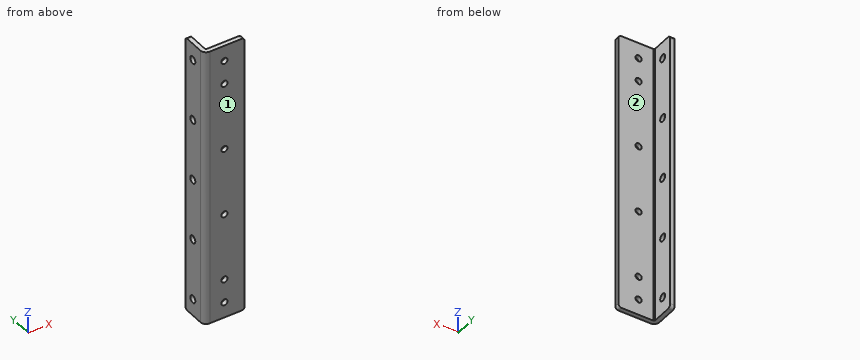
```python
from build123d import *

# Parameters (mm, degrees)
BASE_FLANGE1_START   = -125
BASE_FLANGE1_DEPTH   = 250
FILLET1_R            = 3
M5_CLEARANCE_HOLE1_D = 5.5
M5_CLEARANCE_HOLE2_D = 5.5
M6_CLEARANCE_HOLE1_D = 6.6


# Read off the part's stored shape, not the designer's step: Base-Flange1
with BuildPart() as part:
    # Base-Flange1 outline → Base-Flange1 (new body)
    with BuildSketch(Plane.XY.offset(BASE_FLANGE1_START)):
        with BuildLine():
            Line((5, 0), (36, 0))
            Line((36, 0), (36, 4))
            Line((36, 4), (5, 4))
            ThreePointArc((5, 4), (4.292893219, 4.292893219), (4, 5))
            Line((4, 5), (4, 25))
            Line((4, 25), (0, 25))
            Line((0, 25), (0, 5))
            ThreePointArc((0, 5), (1.464466094, 1.464466094), (5, 0))
        make_face()
    extrude(amount=BASE_FLANGE1_DEPTH)

    # Fillet1
    fillet1_edges = [part.edges().sort_by_distance(p)[0] for p in [
        (2, 25, 125),
        (2, 25, -125),
        (36, 2, 125),
        (36, 2, -125),
    ]]
    fillet(fillet1_edges, radius=FILLET1_R)

    # M5 Clearance Hole1 (through all)
    with Locations(Plane(origin=(0, 4, 0), x_dir=(1, 0, 0), z_dir=(0, 1, 0))):
        with Locations((18, 90), (18, 30), (18, -30), (18, -90)):
            Hole(M5_CLEARANCE_HOLE1_D / 2)

    # M5 Clearance Hole2 (through all)
    with Locations(Plane(origin=(0, 4, 0), x_dir=(1, 0, 0), z_dir=(0, 1, 0))):
        with Locations((18, -111), (18, 111)):
            Hole(M5_CLEARANCE_HOLE2_D / 2)

    # M6 Clearance Hole1 (through all)
    with Locations(Plane(origin=(4, 0, 0), x_dir=(0, 0, -1), z_dir=(1, 0, 0))):
        with Locations((-110, 15), (-55, 15), (0, 15), (55, 15), (110, 15)):
            Hole(M6_CLEARANCE_HOLE1_D / 2)


solid = part.part
```
Design review of the part built by this model. Coordinates are the model's own, in mm. Face numbers are marked on the shaded views. A direction names the side the tool comes from. Coordinates: 2 decimals unless noted, no trailing zeros. Order: outer loops, then holes, each group sorted by start corner. A loop starts at its lowest first (then second) coordinate and runs counter-clockwise, first axis right, second up. Notation, with made-up numbers: (58.25, 39.5) -> (67.25, 39.5) arc R20 cw to (67.25, 58.5) -> close; hole circle Ø4 at (5, -5.75). An arc over 180 degrees is marked (long way). One line per item, written item: value. Start each with the question number.
Q1. Take a section at B-B, the plane x = 18. State the section outline as (y, z) points.
Q2. For probe 1 along Z at (x, y) = (3, 12.5); probe 2 along Y at (x, z) = (32, -0.5); probe 3 along X at (y, z) = (3.5, 92.5), list the stretches that pass through material, from the lowest coordinate up.
Q3. Tool access review of the marked faces 1 and 2: name each direction out of +Z, -Z, +X, -X, +Y, -Y from which nothing blocks a thin tool from reaching the whole face with its end or side.
Q4. Take a section at A-A, the plane z = -30. State the section outline as (x, y) points, then the cut area to 3 significant figures.
Q5. Insertion check: pin 1 Ø7.5 at (y, z) = (15, -110) entering from +X; pin 2 Ø6 at (y, z) = (15, 55) entering from +X; pin 3 Ø7 at (x, z) = (18, -30) entering from -Y; pin 4 Ø9 at (x, z) = (18, -111) entering from +Y. Each pin has a flat end and moves straight along its axis. Give the tip position at first contact, or say it passes through.
Q6. Take a section at C-C, the plane z = 43. State the section outline as (x, y) points.
Q7. Take a section at D-D, the plane z = 111. State the section outline as (x, y) points, then the cut area to 3 significant figures.
Values follow:
1. outline: (0, -125) -> (4, -125) -> (4, -113.75) -> (0, -113.75) -> close; (0, -108.25) -> (4, -108.25) -> (4, -92.75) -> (0, -92.75) -> close; (0, -87.25) -> (4, -87.25) -> (4, -32.75) -> (0, -32.75) -> close; (0, -27.25) -> (4, -27.25) -> (4, 27.25) -> (0, 27.25) -> close; (0, 32.75) -> (4, 32.75) -> (4, 87.25) -> (0, 87.25) -> close; (0, 92.75) -> (4, 92.75) -> (4, 108.25) -> (0, 108.25) -> close; (0, 113.75) -> (4, 113.75) -> (4, 125) -> (0, 125) -> close
2. probe 1: z = -125 to -112.15, -107.85 to -57.15, -52.85 to -2.15, 2.15 to 52.85, 57.15 to 107.85, 112.15 to 125
2. probe 2: y = 0 to 4
2. probe 3: x = 0.23 to 16.85, 19.15 to 36
3. face 1: +Z, -Z, +X, -X, -Y
3. face 2: +Z, -Z, +X, +Y
4. outline: (0, 5) arc R5 ccw to (5, 0) -> (15.25, 0) -> (15.25, 4) -> (5, 4) arc R1 cw to (4, 5) -> (4, 25) -> (0, 25) -> close; (20.75, 0) -> (36, 0) -> (36, 4) -> (20.75, 4) -> close
4. area: 201 mm2
5. pin 1: stops at x = 4
5. pin 2: passes through
5. pin 3: stops at y = 0
5. pin 4: stops at y = 4
6. outline: (0, 5) arc R5 ccw to (5, 0) -> (36, 0) -> (36, 4) -> (5, 4) arc R1 cw to (4, 5) -> (4, 25) -> (0, 25) -> close
7. outline: (0, 5) arc R5 ccw to (5, 0) -> (15.25, 0) -> (15.25, 4) -> (5, 4) arc R1 cw to (4, 5) -> (4, 11.86) -> (0, 11.86) -> close; (0, 18.14) -> (4, 18.14) -> (4, 25) -> (0, 25) -> close; (20.75, 0) -> (36, 0) -> (36, 4) -> (20.75, 4) -> close
7. area: 176 mm2
